Could you check a few things on this model? Use its own coordinates, in mm. Give positions to 0.01 mm unless a question says otherwise; leave off trailing zeros. One line per item, written item: value. Start each with the question number.
Q1. If I drill on line 1 (X direction, y = -185.5, z = 1.9); line 2 (X direction, y = -185, z = 0.35); line 3 (X direction, y = -181, z = 1.2), over which ranges is the centre line in solid material (lowest first)? Write a range as from..to.
Q2. I'm going to push flat-ended pins straight in: P1, Ø1.6, axis at y = -159.5, z = 2, coming from the -X side; P2, Ø6.5, axis at x = 220.11, y = -182.1, coming from the +Z side (3 decimals); P3, Ø1, axis at y = -159.5, z = 2.5, coming from the +X side; P4, Ø1, axis at x = 260.5, z = 2, coming from the -Y side. Where does each tip first touch, or does it pass through?
Q3. I want a section at A-A (z = 0.8). Count the separate pieces of the cut face and the enclosed holes in it, then the cut area to 3 significant figures.
```python
from build123d import *

# Parameters (mm, degrees)
BOSS_EXTRUDE1_DEPTH = 3.175
SKETCH4_R           = 2.1
SKETCH4_R_2         = 2.25
SKETCH4_R_3         = 2.4
CUT_EXTRUDE2_DEPTH  = 343.045224939


with BuildPart() as part:
    # Sketch2 → Boss-Extrude1 (new body)
    with BuildSketch(Plane.XY):
        with BuildLine():
            Line((-166.376823509, -157.21600002), (-166.376823509, -167.12200002))
            Line((-166.376823509, -167.12200002), (-166.376823509, -168.26500002))
            Line((-166.376823509, -168.26500002), (-167.519823509, -168.26500002))
            Line((-167.519823509, -168.26500002), (-167.519823509, -187.31500002))
            Line((-167.519823509, -187.31500002), (-167.519823509, -193.66500002))
            Line((-167.519823509, -193.66500002), (-166.376823509, -193.66500002))
            Line((-166.376823509, -193.66500002), (-166.376823509, -194.18100002))
            Line((-166.376823509, -194.18100002), (-148.199823509, -194.18100002))
            Line((-148.199823509, -194.18100002), (-148.199823509, -203.71400002))
            Line((-148.199823509, -203.71400002), (255.426176451, -203.71400002))
            Line((255.426176451, -203.71400002), (255.426176451, -194.18100002))
            Line((255.426176451, -194.18100002), (273.603176451, -194.18100002))
            Line((273.603176451, -194.18100002), (273.603176451, -193.66500002))
            Line((273.603176451, -193.66500002), (274.746176451, -193.66500002))
            Line((274.746176451, -193.66500002), (274.746176451, -174.61500002))
            Line((274.746176451, -174.61500002), (274.746176451, -168.26500002))
            Line((274.746176451, -168.26500002), (273.603176451, -168.26500002))
            Line((273.603176451, -168.26500002), (273.603176451, -167.12200002))
            Line((273.603176451, -167.12200002), (273.603176451, -157.21600002))
            Line((273.603176451, -157.21600002), (255.463301471, -157.21600002))
            Line((255.463301471, -157.21600002), (255.463301471, -160.70800002))
            ThreePointArc((255.463301471, -160.70800002), (254.533365501, -162.95306405), (252.288301471, -163.88300002))
            Line((252.288301471, -163.88300002), (242.288301471, -163.88300002))
            ThreePointArc((242.288301471, -163.88300002), (240.04323744, -162.95306405), (239.113301471, -160.70800002))
            Line((239.113301471, -160.70800002), (239.113301471, -157.21600002))
            Line((239.113301471, -157.21600002), (220.538301471, -157.21600002))
            Line((220.538301471, -157.21600002), (220.538301471, -160.70800002))
            ThreePointArc((220.538301471, -160.70800002), (219.608365501, -162.95306405), (217.363301471, -163.88300002))
            Line((217.363301471, -163.88300002), (207.363301471, -163.88300002))
            ThreePointArc((207.363301471, -163.88300002), (205.11823744, -162.95306405), (204.188301471, -160.70800002))
            Line((204.188301471, -160.70800002), (204.188301471, -157.21600002))
            Line((204.188301471, -157.21600002), (175.452051471, -157.21600002))
            Line((175.452051471, -157.21600002), (175.452051471, -160.70800002))
            ThreePointArc((175.452051471, -160.70800002), (174.522115501, -162.95306405), (172.277051471, -163.88300002))
            Line((172.277051471, -163.88300002), (162.277051471, -163.88300002))
            ThreePointArc((162.277051471, -163.88300002), (160.03198744, -162.95306405), (159.102051471, -160.70800002))
            Line((159.102051471, -160.70800002), (159.102051471, -157.21600002))
            Line((159.102051471, -157.21600002), (140.527051471, -157.21600002))
            Line((140.527051471, -157.21600002), (140.527051471, -160.70800002))
            ThreePointArc((140.527051471, -160.70800002), (139.597115501, -162.95306405), (137.352051471, -163.88300002))
            Line((137.352051471, -163.88300002), (127.352051471, -163.88300002))
            ThreePointArc((127.352051471, -163.88300002), (125.10698744, -162.95306405), (124.177051471, -160.70800002))
            Line((124.177051471, -160.70800002), (124.177051471, -157.21600002))
            Line((124.177051471, -157.21600002), (73.849301471, -157.21600002))
            Line((73.849301471, -157.21600002), (73.849301471, -160.70800002))
            ThreePointArc((73.849301471, -160.70800002), (72.919365501, -162.95306405), (70.674301471, -163.88300002))
            Line((70.674301471, -163.88300002), (60.674301471, -163.88300002))
            ThreePointArc((60.674301471, -163.88300002), (58.42923744, -162.95306405), (57.499301471, -160.70800002))
            Line((57.499301471, -160.70800002), (57.499301471, -157.21600002))
            Line((57.499301471, -157.21600002), (38.924301471, -157.21600002))
            Line((38.924301471, -157.21600002), (38.924301471, -160.70800002))
            ThreePointArc((38.924301471, -160.70800002), (37.994365501, -162.95306405), (35.749301471, -163.88300002))
            Line((35.749301471, -163.88300002), (25.749301471, -163.88300002))
            ThreePointArc((25.749301471, -163.88300002), (23.50423744, -162.95306405), (22.574301471, -160.70800002))
            Line((22.574301471, -160.70800002), (22.574301471, -157.21600002))
            Line((22.574301471, -157.21600002), (-6.161948529, -157.21600002))
            Line((-6.161948529, -157.21600002), (-6.161948529, -160.70800002))
            ThreePointArc((-6.161948529, -160.70800002), (-7.091884499, -162.95306405), (-9.336948529, -163.88300002))
            Line((-9.336948529, -163.88300002), (-19.336948529, -163.88300002))
            ThreePointArc((-19.336948529, -163.88300002), (-21.58201256, -162.95306405), (-22.511948529, -160.70800002))
            Line((-22.511948529, -160.70800002), (-22.511948529, -157.21600002))
            Line((-22.511948529, -157.21600002), (-41.086948529, -157.21600002))
            Line((-41.086948529, -157.21600002), (-41.086948529, -160.70800002))
            ThreePointArc((-41.086948529, -160.70800002), (-42.016884499, -162.95306405), (-44.261948529, -163.88300002))
            Line((-44.261948529, -163.88300002), (-54.261948529, -163.88300002))
            ThreePointArc((-54.261948529, -163.88300002), (-56.50701256, -162.95306405), (-57.436948529, -160.70800002))
            Line((-57.436948529, -160.70800002), (-57.436948529, -157.21600002))
            Line((-57.436948529, -157.21600002), (-107.764698529, -157.21600002))
            Line((-107.764698529, -157.21600002), (-107.764698529, -160.70800002))
            ThreePointArc((-107.764698529, -160.70800002), (-108.694634499, -162.95306405), (-110.939698529, -163.88300002))
            Line((-110.939698529, -163.88300002), (-120.939698529, -163.88300002))
            ThreePointArc((-120.939698529, -163.88300002), (-123.18476256, -162.95306405), (-124.114698529, -160.70800002))
            Line((-124.114698529, -160.70800002), (-124.114698529, -157.21600002))
            Line((-124.114698529, -157.21600002), (-142.689698529, -157.21600002))
            Line((-142.689698529, -157.21600002), (-142.689698529, -160.70800002))
            ThreePointArc((-142.689698529, -160.70800002), (-143.619634499, -162.95306405), (-145.864698529, -163.88300002))
            Line((-145.864698529, -163.88300002), (-155.864698529, -163.88300002))
            ThreePointArc((-155.864698529, -163.88300002), (-158.10976256, -162.95306405), (-159.039698529, -160.70800002))
            Line((-159.039698529, -160.70800002), (-159.039698529, -157.21600002))
            Line((-159.039698529, -157.21600002), (-166.376823509, -157.21600002))
        make_face()
    extrude(amount=BOSS_EXTRUDE1_DEPTH)

    # Sketch4 → Cut-Extrude2 (cut, through all)
    with BuildSketch(Plane.XY.offset(3.175)):
        with Locations((220.106176451, -182.10474)):
            Circle(SKETCH4_R)
        with Locations((173.906176451, -182.10474)):
            Circle(SKETCH4_R)
        with Locations((-4.519823509, -183.71400002)):
            Circle(SKETCH4_R_2)
        with Locations((-63.519823509, -183.71400002)):
            Circle(SKETCH4_R_2)
        with Locations((-103.723323529, -182.10474)):
            Circle(SKETCH4_R)
        with Locations((-149.923323529, -182.10474)):
            Circle(SKETCH4_R)
        with Locations((48.318076451, -164.10474)):
            Circle(SKETCH4_R_3)
        with Locations((139.818076451, -197.329197785)):
            Circle(SKETCH4_R_3)
    extrude(amount=-CUT_EXTRUDE2_DEPTH, mode=Mode.SUBTRACT)


solid = part.part
```
Worked answers:
1. line 1: x = -167.52..-64.89, -62.15..-5.89, -3.15..274.75
1. line 2: x = -167.52..-65.37, -61.67..-6.37, -2.67..274.75
1. line 3: x = -167.52..-151.71, -148.14..-105.51, -101.94..172.12, 175.69..218.32, 221.89..274.75
2. P1: stops at x = -166.38
2. P2: stops at z = 3.175
2. P3: stops at x = 273.6
2. P4: stops at y = -194.18
3. separate pieces: 1
3. enclosed holes: 8
3. area: 19,000 mm²
